For this review, take the finished solid that the model builds, in its own axes (mm). A direction names the side the tool comes from. Coordinates: 2 decimals unless noted, no trailing zeros. Write each loop counter-clockwise with the first axis right and the second up, starting at its lowest first coordinate (ties: lowest second). Pieces come first, ordered by that corner, then holes.
Autodesk Inventor part; units mm, degrees
ref_plane "Work Plane1" through (-199, 0, 196) normal (0, 0, 1) x (1, 0, 0)
ref_plane "YZ Plane" through (0, 0, 0) normal (1, 0, 0) x (0, 1, 0)
ref_plane "XZ Plane" through (0, 0, 0) normal (0, 1, 0) x (-1, 0, 0)
sketch "Sketch1" plane through (0, 0, 0) normal (0, 1, 0) x (-1, 0, 0)
  line L0 (0, 0) -> (199, 0)
  line L1 (199, 0) -> (199, 199)
  line L2 (199, 199) -> (0, 199)
  line L3 (0, 199) -> (0, 0)
  dimension "d0" = 199
  dimension "d1" = 199
extrude "Extrusion1" add sketch "Sketch1" along normal blind 9
sketch "Sketch2" plane through (0, 9, 0) normal (0, 1, 0) x (1, 0, 0)
  line L0 (0, 0) -> (-199, 0)
  line L1 (-199, -199) -> (0, -199)
  line L2 (0, 0) -> (-2, 0)
  line L3 (-2, 0) -> (-2, -199)
  line L4 (-2, 0) -> (-21, 0)
  line L5 (-21, 0) -> (-21, -199)
  dimension "d4" = 2
  dimension "d5" = 19
extrude "Extrusion2" add sketch "Sketch2" along normal blind 18
sketch "Sketch4" plane through (-199, 0, 199) normal (0, 0, 1) x (1, 0, 0)
  line L0 (178, 27) -> (197, 27)
  line L1 (197, 27) -> (207, 27)
  line L2 (207, 27) -> (207, 41)
  line L3 (178, 27) -> (163, 27)
  line L4 (163, 27) -> (163, 47)
  line L5 (163, 47) -> (165, 47)
  line L6 (165, 47) -> (165, 41)
  line L7 (165, 41) -> (207, 41)
  dimension "d9" = 10
  dimension "d10" = 14
  dimension "d11" = 15
  dimension "d12" = 20
  dimension "d13" = 2
extrude "Extrusion3" add sketch "Sketch4" against normal blind 199
ref_plane "Work Plane1" through (-199, 0, 196) normal (0, 0, 1) x (1, 0, 0)
sketch "Sketch5" plane through (-199, 0, 196) normal (0, 0, 1) x (1, 0, 0)
  line L0 (165, 41) -> (207, 41)
  line L1 (207, 41) -> (207, 68)
  line L2 (165, 68) -> (165, 41)
  line L3 (176.05, 68) -> (176.05, 64.5)
  line L4 (176.05, 64.5) -> (180.3, 61.2)
  line L5 (195.95, 64.5) -> (191.7, 61.2)
  line L6 (195.95, 64.5) -> (195.95, 68)
  line L7 (195.95, 53) -> (195.95, 54.5)
  line L8 (195.95, 54.5) -> (191.7, 61.2)
  line L9 (176.05, 54.5) -> (180.3, 61.2)
  line L10 (176.05, 53) -> (176.05, 54.5)
  line L11 (195.95, 53) -> (176.05, 53)
  line L12 (207, 68) -> (195.95, 68)
  line L13 (207, 68) -> (195.95, 68)
  line L14 (176.05, 68) -> (165, 68)
  line L15 (15, 41) -> (57, 41)
  line L16 (57, 41) -> (57, 68)
  line L17 (15, 68) -> (15, 41)
  line L18 (26.05, 68) -> (26.05, 64.5)
  line L19 (26.05, 64.5) -> (30.3, 61.2)
  line L20 (45.95, 64.5) -> (41.7, 61.2)
  line L21 (45.95, 64.5) -> (45.95, 68)
  line L22 (45.95, 53) -> (45.95, 54.5)
  line L23 (45.95, 54.5) -> (41.7, 61.2)
  line L24 (26.05, 54.5) -> (30.3, 61.2)
  line L25 (26.05, 53) -> (26.05, 54.5)
  line L26 (45.95, 53) -> (26.05, 53)
  line L27 (57, 68) -> (45.95, 68)
  line L28 (57, 68) -> (45.95, 68)
  line L29 (26.05, 68) -> (15, 68)
  line L30 (0, 9) -> (178, 9)
  point P0 (199, 0)
  point P1 (176.05, 51)
  point P2 (26.05, 51)
  dimension "d17" = 27
  dimension "d18" = 1.5
  dimension "d19" = 1.5
  dimension "d20" = 11.05
  dimension "d32" = 27
  dimension "d33" = 1.5
  dimension "d34" = 1.5
  dimension "d35" = 11.05
  dimension "d56" = 32
extrude "Extrusion4" add sketch "Sketch5" against normal blind 193 contours L2 L14 L3 L4 L9 L10 L11 L7 L8 L5 L6 L12 L1 L0
sketch "Sketch6" plane through (-199, 0, 199) normal (0, 0, 1) x (1, 0, 0)
  line L0 (0, 9) -> (178, 9)
  line L1 (0, 9) -> (22, 9)
  line L2 (22, 9) -> (22, 18)
  line L3 (7.723, 18) -> (0, 18)
  line L4 (0, 18) -> (0, 9)
  line L5 (22, 18) -> (22, 27)
  line L6 (22, 41) -> (7.723, 41)
  line L7 (7.723, 41) -> (7.723, 18)
  line L8 (70, 27) -> (70, 41)
  line L9 (70, 41) -> (22, 41)
  line L10 (54, 9) -> (54, 27)
  line L11 (42, 9) -> (42, 27)
  line L12 (22, 27) -> (42, 27)
  line L13 (54, 27) -> (70, 27)
  line L14 (0, 9) -> (22, 9)
  line L15 (42, 9) -> (54, 9)
  dimension "d29" = 20
  dimension "d55" = 14
  dimension "d57" = 18
extrude "Extrusion5" add sketch "Sketch6" against normal blind 199 contours L4 L3 L7 L6 L9 L8 L13 L10 L0 L11 L12 L5 L2
sketch "Sketch8" plane through (-199, 0, 196) normal (0, 0, 1) x (1, 0, 0)
  line L0 (207, 41) -> (165, 41)
  line L1 (207, 41) -> (207, 68)
  line L2 (207, 68) -> (195.95, 68)
  line L3 (195.95, 68) -> (195.95, 64.5)
  line L4 (195.95, 64.5) -> (191.7, 61.2)
  line L5 (191.7, 61.2) -> (195.95, 54.5)
  line L6 (195.95, 54.5) -> (195.95, 53)
  line L7 (195.95, 53) -> (176.05, 53)
  line L8 (176.05, 53) -> (176.05, 54.5)
  line L9 (176.05, 54.5) -> (180.3, 61.2)
  line L10 (180.3, 61.2) -> (176.05, 64.5)
  line L11 (176.05, 64.5) -> (176.05, 68)
  line L12 (176.05, 68) -> (165, 68)
  line L13 (165, 68) -> (165, 47)
  line L14 (165, 41) -> (165, 47)
  line L15 (7.723, 41) -> (70, 41)
  point P0 (199, 0)
extrude "Extrusion6" add sketch "Sketch5" against normal blind 193 contours L17 L29 L18 L19 L24 L25 L26 L22 L23 L20 L21 L27 L16 L15
sketch "Sketch9" plane through (-199, 0, 199) normal (0, 0, 1) x (1, 0, 0)
  line L0 (70, 41) -> (7.723, 41)
  line L1 (57, 41) -> (62, 41)
  line L2 (62, 41) -> (62, 46)
  line L3 (62, 46) -> (57, 46)
  line L4 (57, 46) -> (57, 41)
  line L5 (15, 41) -> (12, 41)
  line L6 (12, 41) -> (12, 46)
  line L7 (12, 46) -> (15, 46)
  line L8 (15, 46) -> (15, 41)
  dimension "d38" = 5
  dimension "d39" = 3
extrude "Extrusion7" add sketch "Sketch9" against normal blind 199
sketch "Sketch10" plane through (-199, 0, 199) normal (0, 0, 1) x (1, 0, 0)
  line L0 (62, 41) -> (62, 46)
  line L1 (62, 41) -> (70, 41)
  line L2 (70, 68) -> (62, 68)
  line L3 (62, 68) -> (62, 41)
  line L4 (70, 55.5) -> (105, 55.5)
  line L5 (70, 55.5) -> (105, 55.5)
  line L6 (70, 50.5) -> (105, 50.5)
  line L7 (70, 50.5) -> (105, 50.5)
  line L8 (70, 50.5) -> (105, 50.5)
  line L9 (105, 50.5) -> (105, 55.5)
  line L10 (105, 55.5) -> (70, 55.5)
  line L11 (70, 37) -> (70, 50.5)
  line L12 (70, 55.5) -> (70, 68)
  line L13 (70, 41) -> (70, 50.5)
  line L14 (70, 55.5) -> (70, 68)
  point P0 (0, 0)
  dimension "d42" = 35
  dimension "d59" = 27
  dimension "d60" = 12.5
  dimension "d61" = 5
extrude "Extrusion8" add sketch "Sketch10" against normal blind 199
extrude "Extrusion9" add sketch "Sketch10" along normal blind 60
sketch "Sketch11" plane through (-199, 0, 199) normal (0, 0, 1) x (1, 0, 0)
  line L0 (178, 27) -> (183, 27)
  line L1 (183, 27) -> (183, 32)
  circle A0 centre (183, 32) radius 2.5
  dimension "d47" = 5
  dimension "d50" = 5
extrude "Extrusion10" add sketch "Sketch11" along normal blind 55
sketch "Sketch12" plane through (0, 0, 0) normal (0, 0, -1) x (-1, 0, 0)
  circle A0 centre (16, 32) radius 2.5
  circle A1 centre (16, 32) radius 2.5
extrude "Extrusion11" add sketch "Sketch12" along normal blind 55
properties part number "Platform" material "Steel"
Q1. Add section A-A (x = -124.5). State the section outline as (y, z) points, then the cut area to 3 significant figures.
Ans:
outline: (0, 0) - (9, 0) - (9, 199) - (0, 199) - close; (50.5, 0) - (55.5, 0) - (55.5, 259) - (50.5, 259) - close
area: 3,090 mm2
Q2. Clearance check with flat-ended pins moving along their axes: pin 1 Ø6 at (x, z) = (-22.5, 201.5) entering from +Y; pin 2 Ø1.5 at (y, z) = (44.5, 1.5) entering from +X; pin 3 Ø5 at (x, y) = (-157, 21) entering from -Z; pin 4 Ø5 at (x, y) = (-120.5, 12) entering from +Z. State where each tip first meets the part, or that it passes through.
Ans:
pin 1: stops at y = 41
pin 2: stops at x = -34
pin 3: stops at z = 0
pin 4: passes through
Q3. For probe 1 along X at (y, z) = (24, 13); probe 2 along X at (y, z) = (51, 179.5); probe 3 along Y at (x, z) = (-117.5, 111.5), list the stretches that pass through material, from the lowest coordinate up.
Ans:
probe 1: x = -191.28 to -177, -157 to -145, -21 to -2
probe 2: x = -184 to -142, -137 to -94, -34 to 8
probe 3: y = 0 to 9, 50.5 to 55.5
Q4. Tool access review of faces 1 (the flat face through (-195, 18, 101)), 2 (the flat face through (-163, 52, 3)), 3 (the flat face through (-129, 39, 128)), 4 (the flat face through (-163, 52, 196)): name each direction out of +Z, -Z, +X, -X, +Y, -Y from which nothing blocks a thin tool from reaching the whole face with its end or side.
Ans:
face 1: +Z, -Z, -X, +Y
face 2: -Z, +Y
face 3: +Z, -Z
face 4: +Z, +Y
Q5. Add section B-B (z = 212). State the section outline as (x, y) points, then the cut area to 3 significant figures.
Ans:
outline: (-137, 41) - (-129, 41) - (-129, 50.5) - (-94, 50.5) - (-94, 55.5) - (-129, 55.5) - (-129, 68) - (-137, 68) - close; circle Ø5 at (-16, 32)
area: 411 mm2
Q6. Add section C-C (x = -45). State the section outline as (y, z) points, then the cut area to 3 significant figures.
Ans:
outline: (0, 0) - (9, 0) - (9, 199) - (0, 199) - close
area: 1,790 mm2
Q7. Draft analysis for pull direction Y (two halves, no side actions). For faces 5 (the flat face through (-21, 18, 98)), 6 (the flat face through (-133, 41, 229)), 7 (the flat face through (-184, 57, 101)), state which applies: +Y half, -Y half, draft (parallel to the pull), parting line (faces both ways), or undercut.
Ans:
face 5: undercut
face 6: -Y half
face 7: draft
